Source: three-view drawing plus pictorial views. Frame: mm from the lowest corner of the part. A direction names the side the tool comes from. Coordinates: 2 decimals unless noted, no trailing zeros. Loops run counter-clockwise (first coordinate to the right, second up) from the corner with the lowest first, then second, coordinate; pieces in that order, holes last. Notation, with made-up numbers: (21.25, 24) - (28.25, 24) arc R12 ccw to (28.25, 30) - close; hole circle Ø9 at (2.5, 53.5). An arc over 180 degrees is marked (long way). Use CSV: the item, a comma, the result in double quotes. Start each with the question number.
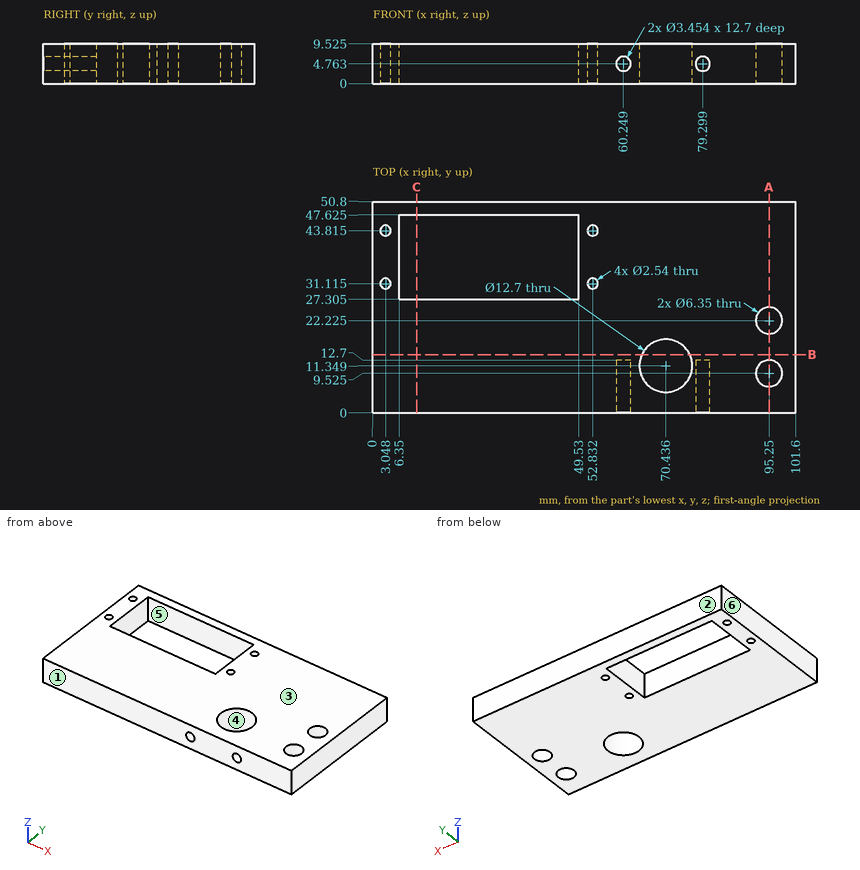
(1) Section B-B on y = 14. Output: boundary loops of the cut face in (x, z) (1 decimal).
(2) Pin query (flat end, axial travel): pin 1 Ø3.5 at (x, y) = (3.048, 31.115) entering from -Z; pin 2 Ø1.7 at (x, z) = (60.5, 5.5) entering from -Y. Return the tip coordinate at first contact, or that it passes through.
(3) Reachability of the marked faces 5 and 6 from +Z, -Z, +X, -X, +Y, -Y: full face, straight path, thin tool, end or side. Return the list, or none.
(4) Section C-C on x = 10.5. Output: boundary loops of the cut face in (y, z) (1 decimal).
(5) Section A-A on x = 95.25. State how many separate pieces and enclosed holes the cut face has, plus the area to 3 significant figures.
(6) Ray query, line 1 (Y direction, x = 46, z = 8.25) (1 decimal); line 2 (X direction, y = 33.5, z = 9.25); line 3 (Y direction, x = 96, z = 4.25). Return the intervals inside material, ascending. Write a range as [from, to].
(7) Draft query along Y for the marked faces 1, 2, 3 and 4. Return one class per face: released by +Y, released by -Y, zero draft, split by the parting line, or undercut.
Solution:
1,outline,"(0, 0) - (64.7, 0) - (64.7, 9.5) - (0, 9.5) - close; (76.2, 0) - (101.6, 0) - (101.6, 9.5) - (76.2, 9.5) - close"
2,pin 1,"stops at z = 0"
2,pin 2,"stops at y = 12.7"
3,face 5,"+Z, -Z"
3,face 6,"+Z, -Z, -X, +Y, -Y"
4,outline,"(0, 0) - (27.3, 0) - (27.3, 9.5) - (0, 9.5) - close; (47.6, 0) - (50.8, 0) - (50.8, 9.5) - (47.6, 9.5) - close"
5,separate pieces,"3"
5,enclosed holes,"0"
5,area,"363 mm²"
6,line 1,"y = [0, 27.3], [47.6, 50.8]"
6,line 2,"x = [0, 6.35], [49.53, 101.6]"
6,line 3,"y = [0, 6.44], [12.61, 19.14], [25.31, 50.8]"
7,face 1,"released by -Y"
7,face 2,"released by +Y"
7,face 3,"zero draft"
7,face 4,"undercut"
